```python
from build123d import *

# Parameters (mm, degrees)
BOSS_EXTRUDE1_DEPTH     = 50
BOSS_EXTRUDE2_DEPTH     = 50
CUT_EXTRUDE1_DEPTH      = 56.88006898
CUT_EXTRUDE1_DEPTH_BACK = 56.88006898
SKETCH3_W               = 15
SKETCH3_H               = 0.75
FILLET1_DEPTH           = 50
FILLET2_DEPTH           = 50
FILLET3_R               = 1


with BuildPart() as part:
    # Sketch1 → Boss-Extrude1 (new body)
    with BuildSketch(Plane.XY):
        Polygon((-4, -2), (16.92820323, -2), (16.92820323, -1.053536475), (-1.931851653, 4), (16.92820323, 9.053536475), (16.92820323, 10), (-4, 10), align=None)
    extrude(amount=BOSS_EXTRUDE1_DEPTH)

    # Sketch2 → Boss-Extrude2 (add)
    with BuildSketch(Plane.XY.offset(50)):
        Polygon((-5.931851653, 4), (-4, 10), (-4, -2), align=None)
    extrude(amount=-BOSS_EXTRUDE2_DEPTH)

    # Sketch3 → Cut-Extrude1 (cut, two sides: drawn at the far end of the back side and taken through both)
    with BuildSketch(Plane(origin=(-5.931851653, 0, 0), x_dir=(0, 0, -1), z_dir=(1, 0, 0)).offset(-CUT_EXTRUDE1_DEPTH_BACK)):
        with Locations((-25, 3.625)):
            Rectangle(SKETCH3_W, SKETCH3_H)
        with Locations((-25, 4.375)):
            Rectangle(SKETCH3_W, SKETCH3_H)
    extrude(amount=CUT_EXTRUDE1_DEPTH + CUT_EXTRUDE1_DEPTH_BACK, mode=Mode.SUBTRACT)

    # Fillet1: read off the stored shape, not the designer's step
    # Fillet1 outline → Fillet1 (cut)
    with BuildSketch(Plane.XY):
        with BuildLine():
            ThreePointArc((-5.931851653, 4), (-2.243925838, 8.366600265), (3.233299737, 10))
            Line((3.233299737, 10), (-4, 10))
            Line((-4, 10), (-5.931851653, 4))
        make_face()
    extrude(amount=FILLET1_DEPTH, mode=Mode.SUBTRACT)

    # Fillet2: read off the stored shape, not the designer's step
    # Fillet2 outline → Fillet2 (cut)
    with BuildSketch(Plane.XY):
        with BuildLine():
            ThreePointArc((3.233299737, -2), (-2.243925838, -0.366600265), (-5.931851653, 4))
            Line((-5.931851653, 4), (-4, -2))
            Line((-4, -2), (3.233299737, -2))
        make_face()
    extrude(amount=FILLET2_DEPTH, mode=Mode.SUBTRACT)

    # Fillet3
    fillet3_edges = [part.edges().sort_by_distance(p)[0] for p in [
        (16.92820323, -1.053536475, 25),
        (16.92820323, 9.053536475, 25),
    ]]
    fillet(fillet3_edges, radius=FILLET3_R)


solid = part.part
```
Geometry: final body of the model. Coordinates: model frame, mm. A direction names the side the tool comes from. Round coordinates to 2 decimals unless told otherwise and drop trailing zeros. Loops run counter-clockwise (first coordinate to the right, second up) from the corner with the lowest first, then second, coordinate; pieces in that order, holes last. Notation, with made-up numbers: (-29, -21) -> (8, -21) arc R31 cw to (8, 12) -> close; hole circle Ø3 at (61.5, 13). An arc over 180 degrees is marked (long way). Use one line per item in the form item = value. Start each with the question number.
1) Section A-A on z = 20. Output: boundary loops of the cut face in (x, y).
2) Access query for faces 4 (the cylindrical face through (-2.312, 8.322, 24.65)), 5 (the flat face through (-3, 4, 32.5)), 6 (the cylindrical face through (16.73, -1.22, 25.35)). Directions: +Z, -Z, +X, -X, +Y, -Y. A direction counts if a zero-diameter tool reaches every point of the face in a straight line with its end or side. Return the directions, or none.
3) First-contact query: P1, Ø6, axis at x = 6.5, y = 5, coming from the +Z side; P2, Ø10, axis at x = -3.5, z = 19.5, coming from the -Y side; P3, Ø1.9, axis at x = -2, z = 23.5, coming from the +Y side; P4, Ø1.9, axis at x = -3, z = 27, coming from the -Y side. Flat tips, straight axial feed; report the tip coordinate or a pass-through.
4) Draft query along Y for faces 1 (the cylindrical face through (16.716, 9.205, 25.35)), 2 (the flat face through (3, 7, 50)), 3 (the flat face through (10, -2, 25)). Return one class per face: released by +Y, released by -Y, zero draft, split by the parting line, or undercut.
5) Section B-B on x = 8.5. Output: boundary loops of the cut face in (y, z), then the cut area to 3 significant figures.
6) Section D-D on x = -0.25. Output: boundary loops of the cut face in (y, z), then the cut area to 3 significant figures.
7) Section C-C on x = -3.5. Output: boundary loops of the cut face in (y, z).
8) Line query: L1, parallel to Y at x = 12, z = 46; L2, parallel to Y at x = 12.75, z = 47; L3, parallel to X at y = 9, z = 28. Output: solid intervals per line, ascending.
Response:
q1.outline = (-5.57, 3.25) arc R10 ccw to (3.23, -2) -> (16.93, -2) -> (16.93, -1.82) arc R1 ccw to (16.19, -0.85) -> (0.87, 3.25) -> close; (-5.57, 4.75) -> (0.87, 4.75) -> (16.19, 8.85) arc R1 ccw to (16.93, 9.82) -> (16.93, 10) -> (3.23, 10) arc R10 ccw to start
q2.face_4 = +Z, -Z, -X, +Y
q2.face_5 = +X, -X
q2.face_6 = +Z, -Z, +X
q3.P1 = 50
q3.P2 = -1.85
q3.P3 = 9.04
q3.P4 = -0.49
q4.face_1 = undercut
q4.face_2 = zero draft
q4.face_3 = released by -Y
q5.outline = (-2, 0) -> (1.2, 0) -> (1.2, 50) -> (-2, 50) -> close; (6.8, 0) -> (10, 0) -> (10, 50) -> (6.8, 50) -> close
q5.area = 320 mm^2
q6.outline = (-1.37, 0) -> (3.55, 0) -> (3.55, 17.5) -> (3.25, 17.5) -> (3.25, 32.5) -> (3.55, 32.5) -> (3.55, 50) -> (-1.37, 50) -> close; (4.45, 0) -> (9.37, 0) -> (9.37, 50) -> (4.45, 50) -> (4.45, 32.5) -> (4.75, 32.5) -> (4.75, 17.5) -> (4.45, 17.5) -> close
q6.area = 483 mm^2
q7.outline = (0.61, 0) -> (7.39, 0) -> (7.39, 50) -> (0.61, 50) -> close; hole (3.25, 17.5) -> (4.75, 17.5) -> (4.75, 32.5) -> (3.25, 32.5) -> close
q8.L1 = -2 to 0.27, 7.73 to 10
q8.L2 = -2 to 0.07, 7.93 to 10
q8.L3 = -1.13 to 16.5
